from build123d import *

# Parameters (mm, degrees)
CUT_EXTRUDE_1_DEPTH = 3
CUT_EXTRUDE_2_DEPTH = 1.8


with BuildPart() as part:
    # 草图1 → 旋转1 (revolve)
    with BuildSketch(Plane.XY, mode=Mode.PRIVATE) as revolve_1_sk:
        Polygon((0, 0), (0, 4), (8, 4), (8, 5), (14, 5), (14, 6), (26, 6), (26, 5), (32, 5), (32, 4), (40, 4), (40, 0), align=None)
    revolve(revolve_1_sk.sketch.rotate(Axis((0, 0, 0), (1, 0, 0)), 180), axis=Axis((0, 0, 0), (1, 0, 0)))

    # 草图2 → 切除-拉伸1 (cut)
    with BuildSketch(Plane.XY.offset(6)):
        with BuildLine():
            Line((17.5, 2.5), (22.5, 2.5))
            ThreePointArc((22.5, 2.5), (25, 0), (22.5, -2.5))
            Line((22.5, -2.5), (17.5, -2.5))
            ThreePointArc((17.5, -2.5), (15, 0), (17.5, 2.5))
        make_face()
    extrude(amount=-CUT_EXTRUDE_1_DEPTH, mode=Mode.SUBTRACT)

    # 草图3 → 切除-拉伸2 (cut)
    with BuildSketch(Plane.XY.offset(4)):
        with BuildLine():
            Line((2.5, 1.5), (5.5, 1.5))
            ThreePointArc((5.5, 1.5), (7, 0), (5.5, -1.5))
            Line((5.5, -1.5), (2.5, -1.5))
            ThreePointArc((2.5, -1.5), (1, 0), (2.5, 1.5))
        make_face()
        with BuildLine():
            Line((37.5, 1.5), (34.5, 1.5))
            ThreePointArc((34.5, 1.5), (33, 0), (34.5, -1.5))
            Line((34.5, -1.5), (37.5, -1.5))
            ThreePointArc((37.5, -1.5), (39, 0), (37.5, 1.5))
        make_face()
    cut_extrude_2 = extrude(amount=-CUT_EXTRUDE_2_DEPTH, mode=Mode.SUBTRACT)

    # 镜向1: 切除-拉伸2 across plane
    add(cut_extrude_2.mirror(Plane.XY), mode=Mode.SUBTRACT)


solid = part.part
Part model, mm, in its own coordinate system. A direction names the side the tool comes from. Give positions to 0.01 mm unless a question says otherwise; leave off trailing zeros. Order: outer loops, then holes, each group sorted by start corner. A loop starts at its lowest first (then second) coordinate and runs counter-clockwise, first axis right, second up. Notation, with made-up numbers: (43, -17.75) -> (100, -17.75) arc R20 ccw to (100, 21.25) -> close; hole circle Ø3 at (-38, 27). An arc over 180 degrees is marked (long way). Use one line per item in the form item = value.
(1) Pull direction Y, two halves, no side cores. Call faces 5 (the face through (26, 4, -4)), 6 (the face through (4, 0, 2.2)), 7 (the face through (20.084, -3.226, -5.059)): +Y half, -Y half, draft (parallel to the pull), parting line (faces both ways), or undercut.
Solution:
face_5 = draft
face_6 = undercut
face_7 = parting line
(2) Saw through at B-B (x = 3). Write the cut outline in (y, z).
Solution:
outline = (-1.5, -3.71) -> (-1.5, -2.2) -> (1.5, -2.2) -> (1.5, -3.71) arc R4 ccw to (1.5, 3.71) -> (1.5, 2.2) -> (-1.5, 2.2) -> (-1.5, 3.71) arc R4 ccw to start
(3) Tool access for faces 1 (the face through (11, 5, 0)), 2 (the face through (36, -1.5, 3)), 3 (the face through (36.056, -3.815, -1.201)), 4 (the face through (4, -1.5, -3)): list every direction of +Z, -Z, +X, -X, +Y, -Y with a clear straight run to the whole face (end or side of a thin tool).
Solution:
face_1 = -X
face_2 = +Z
face_3 = +X
face_4 = -Z
(4) Flat gauge pins, fed straight in: P1, Ø0.8, axis at x = 4.5, z = -3.5, coming from the -Y side; P2, Ø3, axis at x = 26.5, y = -3.5, coming from the -Z side; P3, Ø1.5, axis at x = 5.5, z = -2, coming from the -Y side; P4, Ø4, axis at y = 4, z = -2, coming from the +X side. Where does each tip first touch, or does it go through?
Solution:
P1 = -2.53
P2 = -5.63
P3 = -3.8
P4 = 40
(5) Saw through at A-A (z = 0). Write the cut outline in (x, y).
Solution:
outline = (0, -4) -> (8, -4) -> (8, -5) -> (14, -5) -> (14, -6) -> (26, -6) -> (26, -5) -> (32, -5) -> (32, -4) -> (40, -4) -> (40, 4) -> (32, 4) -> (32, 5) -> (26, 5) -> (26, 6) -> (14, 6) -> (14, 5) -> (8, 5) -> (8, 4) -> (0, 4) -> close
(6) Drill centre lines: line 1 (X direction, y = -4, z = -1); line 2 (Y direction, x = 20, z = -0.25); line 3 (X direction, y = -5, z = -3). Where is each one in solid material? Low to high. Write a range as from..to.
Solution:
line_1 = 8..32
line_2 = -5.99..5.99
line_3 = 14..26
(7) Saw through at C-C (y = -3). Write the cut outline in (x, z), then the cut area to 3 significant figures.
Solution:
outline = (0, -2.65) -> (8, -2.65) -> (8, -4) -> (14, -4) -> (14, -5.2) -> (26, -5.2) -> (26, -4) -> (32, -4) -> (32, -2.65) -> (40, -2.65) -> (40, 2.65) -> (32, 2.65) -> (32, 4) -> (26, 4) -> (26, 5.2) -> (14, 5.2) -> (14, 4) -> (8, 4) -> (8, 2.65) -> (0, 2.65) -> close
area = 305 mm²
(8) Saw through at D-D (x = 25.5). Write the cut outline in (y, z).
Solution:
outline = circle Ø12 at (0, 0)
